Part model, mm, in its own coordinate system. A direction names the side the tool comes from. Coordinates: 2 decimals unless noted, no trailing zeros. Order: outer loops, then holes, each group sorted by start corner. A loop starts at its lowest first (then second) coordinate and runs counter-clockwise, first axis right, second up. Notation, with made-up numbers: (8, -14) - (40, -14) arc R22 ccw to (40, -2) - close; hole circle Ø2 at (21.25, -8.5). An arc over 180 degrees is marked (long way). Use a Markdown table: item, result. Add a question column.
1) Saw through at B-B on z = -6.25. List the corners of the cut face in (x, y).
2) Tool access for faces 5 (the face through (-30, 20, 5)), 6 (the face through (-45.41, 2.03, -7.69)), 7 (the face through (-30, 14, 3.111)), 8 (the face through (-29, 7.797, 5)): list every direction of +Z, -Z, +X, -X, +Y, -Y with a clear straight run to the whole face (end or side of a thin tool).
3) Saw through at D-D on z = 4. List the corners of the cut face in (x, y), then the cut area to 3 significant figures.
4) Saw through at A-A on x = -32. List the corners of the cut face in (y, z), then the cut area to 3 significant figures.
5) Two-plate mould, pull along X, no slides. Class faces 1 (the face through (-29, 2, -5.589)), 2 (the face through (-49.259, 3, 2)), 3 (the face through (-30, 2, -12.889)), 4 (the face through (-9.259, 3, 2)): +X half, -X half, draft (parallel to the pull), parting line (faces both ways), or undercut.
6) Wall check: L1, parallel to Y at x = -34, z = 5.75; L2, parallel to Z at x = -30, y = 4.25; L3, parallel to Y at x = -46.5, z = -0.5. Give the ranges that are in metal, low to high. Write a range as [from, to].
7) Drop a flat-ended pin along its axis: P1, Ø1, axis at x = -14.5, z = -0.5, coming from the +Y side. Give the stop position or say it passes through.
8) Saw through at C-C on y = 8.25. List the corners of the cut face in (x, z), then the cut area to 3 significant figures.
```python
from build123d import *

# Parameters (mm, degrees)
SKETCH1_W           = 40
SKETCH1_H           = 20
BOSS_EXTRUDE1_DEPTH = 4
SKETCH5_W           = 40
SKETCH5_H           = 4
BOSS_EXTRUDE2_DEPTH = 16
CUT_EXTRUDE3_DEPTH  = 10
CUT_EXTRUDE5_DEPTH  = 10


with BuildPart() as part:
    # Sketch1 → Boss-Extrude1 (new body)
    with BuildSketch(Plane(origin=(0, 0, 0), x_dir=(1, 0, 0), z_dir=(0, 1, 0))):
        with Locations((-29.259259259, 2.888888889)):
            Rectangle(SKETCH1_W, SKETCH1_H)
    extrude(amount=BOSS_EXTRUDE1_DEPTH)

    # Sketch5 → Boss-Extrude2 (add)
    with BuildSketch(Plane(origin=(0, 4, 0), x_dir=(1, 0, 0), z_dir=(0, 1, 0))):
        with Locations((-29.259259259, -5.111111111)):
            Rectangle(SKETCH5_W, SKETCH5_H)
    extrude(amount=BOSS_EXTRUDE2_DEPTH)

    # Sketch7 → Cut-Extrude3 (cut)
    with BuildSketch(Plane(origin=(0, 4, 0), x_dir=(1, 0, 0), z_dir=(0, 1, 0))):
        with BuildLine():
            Line((-15.259259259, 5.588888889), (-43.259259259, 5.588888889))
            ThreePointArc((-43.259259259, 5.588888889), (-45.409259259, 7.738888889), (-43.259259259, 9.888888889))
            Line((-43.259259259, 9.888888889), (-15.259259259, 9.888888889))
            ThreePointArc((-15.259259259, 9.888888889), (-13.109259259, 7.738888889), (-15.259259259, 5.588888889))
        make_face()
    extrude(amount=-CUT_EXTRUDE3_DEPTH, mode=Mode.SUBTRACT)

    # Sketch8 → Cut-Extrude5 (cut)
    with BuildSketch(Plane(origin=(0, 0, 3.111111111), x_dir=(-1, 0, 0), z_dir=(0, 0, -1))):
        with BuildLine():
            Line((24.259259259, 11.997218425), (34.259259259, 11.997218425))
            ThreePointArc((34.259259259, 11.997218425), (36.359259259, 9.897218425), (34.259259259, 7.797218425))
            Line((34.259259259, 7.797218425), (24.259259259, 7.797218425))
            ThreePointArc((24.259259259, 7.797218425), (22.159259259, 9.897218425), (24.259259259, 11.997218425))
        make_face()
    extrude(amount=-CUT_EXTRUDE5_DEPTH, mode=Mode.SUBTRACT)


solid = part.part
```
Results are:
| question | item | result |
|---|---|---|
| 1 | outline | (-49.26, 0) - (-44.81, 0) - (-44.81, 4) - (-49.26, 4) - close; (-13.71, 0) - (-9.26, 0) - (-9.26, 4) - (-13.71, 4) - close |
| 2 | face 5 | +Z, -Z, +X, -X, +Y |
| 2 | face 6 | +Y, -Y |
| 2 | face 7 | -Z, +X, -X, +Y |
| 2 | face 8 | +Z, -Z |
| 3 | outline | (-49.26, 0) - (-9.26, 0) - (-9.26, 20) - (-49.26, 20) - close; hole (-34.26, 7.8) - (-24.26, 7.8) arc R2.1 ccw to (-24.26, 12) - (-34.26, 12) arc R2.1 ccw to start |
| 3 | area | 744 mm2 |
| 4 | outline | (0, -12.89) - (4, -12.89) - (4, -9.89) - (0, -9.89) - close; (0, -5.59) - (4, -5.59) - (4, 3.11) - (7.8, 3.11) - (7.8, 7.11) - (0, 7.11) - close; (12, 3.11) - (20, 3.11) - (20, 7.11) - (12, 7.11) - close |
| 4 | area | 110 mm2 |
| 5 | face 1 | undercut |
| 5 | face 2 | -X half |
| 5 | face 3 | draft |
| 5 | face 4 | +X half |
| 6 | L1 | [0, 7.8], [12, 20] |
| 6 | L2 | [3.11, 7.11] |
| 6 | L3 | [0, 4] |
| 7 | P1 | y = 4 |
| 8 | outline | (-49.26, 3.11) - (-35.56, 3.11) - (-35.56, 7.11) - (-49.26, 7.11) - close; (-22.96, 3.11) - (-9.26, 3.11) - (-9.26, 7.11) - (-22.96, 7.11) - close |
| 8 | area | 110 mm2 |
